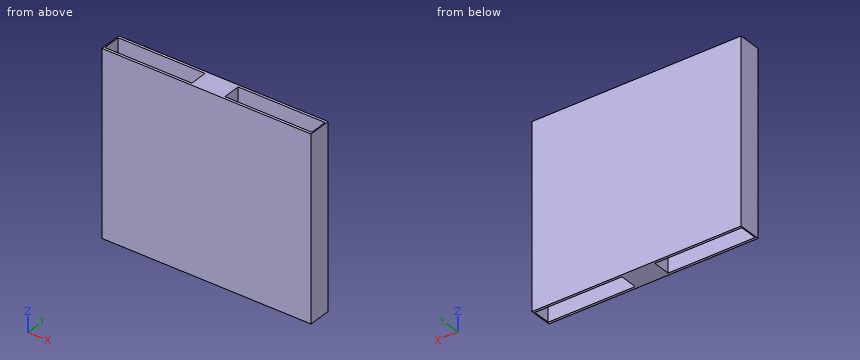
from build123d import *

# Parameters (mm, degrees)
CROQUIS1_W              = 1200
CROQUIS1_H              = 800
SALIENTE_EXTRUIR1_DEPTH = 100
CROQUIS2_W              = 382.5
CROQUIS2_H              = 78
CORTAR_EXTRUIR2_DEPTH   = 1446.68322948
CROQUIS3_W              = 140.2375
CROQUIS3_H              = 100
CORTAR_EXTRUIR3_DEPTH   = 1446.68322948


with BuildPart() as part:
    # Croquis1 → Saliente-Extruir1 (new body)
    with BuildSketch(Plane(origin=(0, 0, 0), x_dir=(1, 0, 0), z_dir=(0, 1, 0))):
        with Locations((600, 400)):
            Rectangle(CROQUIS1_W, CROQUIS1_H)
    extrude(amount=SALIENTE_EXTRUIR1_DEPTH)

    # Croquis2 → Cortar-Extruir2 (cut, through all)
    with BuildSketch(Plane.XY):
        with Locations((336.25, 50)):
            Rectangle(CROQUIS2_W, CROQUIS2_H)
        with Locations((863.75, 50)):
            Rectangle(CROQUIS2_W, CROQUIS2_H)
    extrude(amount=-CORTAR_EXTRUIR2_DEPTH, mode=Mode.SUBTRACT)

    # Croquis3 → Cortar-Extruir3 (cut, through all)
    with BuildSketch(Plane.XY):
        with Locations((70.11875, 50)):
            Rectangle(CROQUIS3_W, CROQUIS3_H)
        with Locations((1129.88125, 50)):
            Rectangle(CROQUIS3_W, CROQUIS3_H)
    extrude(amount=-CORTAR_EXTRUIR3_DEPTH, mode=Mode.SUBTRACT)


solid = part.part
Input: part model. Units: mm. Frame: model coordinates. Give positions to 0.01 mm unless a question says otherwise; leave off trailing zeros. Write each loop counter-clockwise with the first axis right and the second up, starting at its lowest first coordinate (ties: lowest second). Pieces come first, ordered by that corner, then holes.
Q1. Material intervals for probe 1 along X at (y, z) = (23, -751); probe 2 along Y at (x, z) = (797, -646.5), sorted ascending.
Q2. Section B-B, the plane x = 926. Output: boundary loops of the cut face in (y, z), plus the area to 3 significant figures.
Q3. Section A-A, the plane y = 27.5. Output: boundary loops of the cut face in (x, z).
Q4. First-contact query: P1, Ø12, axis at x = 426, z = -423.5, coming from the -Y side. Flat tip, straight axial feed; report the tip coordinate or a pass-through.
Q5. Section C-C, the plane z = -538. Output: boundary loops of the cut face in (x, y).
Filled in:
1. probe 1: x = 140.24 to 145, 527.5 to 672.5, 1055 to 1059.76
1. probe 2: y = 0 to 11, 89 to 100
2. outline: (0, -800) - (11, -800) - (11, 0) - (0, 0) - close; (89, -800) - (100, -800) - (100, 0) - (89, 0) - close
2. area: 17,600 mm2
3. outline: (140.24, -800) - (145, -800) - (145, 0) - (140.24, 0) - close; (527.5, -800) - (672.5, -800) - (672.5, 0) - (527.5, 0) - close; (1055, -800) - (1059.76, -800) - (1059.76, 0) - (1055, 0) - close
4. P1: stops at y = 0
5. outline: (140.24, 0) - (1059.76, 0) - (1059.76, 100) - (140.24, 100) - close; hole (145, 11) - (527.5, 11) - (527.5, 89) - (145, 89) - close; hole (672.5, 11) - (1055, 11) - (1055, 89) - (672.5, 89) - close
